The model under review builds one solid part; all positions refer to its coordinate system, in mm. Face numbers are marked on the shaded views. A direction names the side the tool comes from. Give positions to 0.01 mm unless a question says otherwise; leave off trailing zeros. Order: outer loops, then holes, each group sorted by start corner. A loop starts at its lowest first (then second) coordinate and runs counter-clockwise, first axis right, second up.
```python
from build123d import *

# Parameters (mm, degrees)
EXTRUDE_1_DEPTH             = 25
CHAMFER_5_SIZE              = 2.5
SKETCH_6_W                  = 20.2
SKETCH_6_H                  = 41.891303575
CUT_EXTRUDE_2_DEPTH         = 7.6
SKETCH_7_R                  = 5.25
SKETCH_7_R_2                = 4.1
CUT_EXTRUDE_3_DEPTH         = 76.352903063
SKETCH_8_W                  = 20.2
SKETCH_8_H                  = 8.585894888
CUT_EXTRUDE_4_DEPTH         = 5.1
FILLET_2_R                  = 2
CUT_EXTRUDE_5_REACH         = 77.353
SKETCH_10_R                 = 1.5
M3X0_51_D                   = 2.5
M3X0_51_DEPTH               = 3
M3X0_51_TIP                 = 0.751075774
EXTRUDE_3_DEPTH             = 5
FILLET_3_R                  = 2
HOLE_WIZARD_M32_D           = 3.4
HOLE_WIZARD_M32_CBORE_D     = 6.5
HOLE_WIZARD_M32_CBORE_DEPTH = 2.5


with BuildPart() as part:
    # Эскиз1 → Бобышка-Вытянуть1 (new body)
    with BuildSketch(Plane.XY):
        with BuildLine():
            Line((0, 0), (0, 70.5))
            Line((0, 70.5), (-3.6, 70.5))
            ThreePointArc((-3.6, 70.5), (-7.489087297, 68.889087297), (-9.1, 65))
            Line((-9.1, 65), (-9.1, 32))
            ThreePointArc((-9.1, 32), (-8.15059166, 22.302605618), (-5.338421688, 12.97348272))
            Line((-5.338421688, 12.97348272), (0, 0))
        make_face()
    extrude(amount=EXTRUDE_1_DEPTH)

    # Фаска5
    chamfer_5_edges = [part.edges().sort_by_distance(p)[0] for p in [
        (-8.15059166, 22.302605618, 25),
        (-2.669210844, 6.48674136, 25),
        (-1.8, 70.5, 25),
        (-7.489087297, 68.889087297, 25),
        (-1.8, 70.5, 0),
        (-2.669210844, 6.48674136, 0),
        (-9.1, 48.5, 25),
        (-8.15059166, 22.302605618, 0),
        (-9.1, 48.5, 0),
        (-7.489087297, 68.889087297, 0),
    ]]
    chamfer(chamfer_5_edges, length=CHAMFER_5_SIZE)

    # Эскиз6 → Вырез-Вытянуть2 (cut)
    with BuildSketch(Plane(origin=(0, 0, 0), x_dir=(0, 0, -1), z_dir=(1, 0, 0))):
        with Locations((-12.5, 46.054348213)):
            Rectangle(SKETCH_6_W, SKETCH_6_H)
    extrude(amount=-CUT_EXTRUDE_2_DEPTH, mode=Mode.SUBTRACT)

    # Эскиз7 → Вырез-Вытянуть3 (cut, through all)
    with BuildSketch(Plane.ZY.offset(9.1)):
        with Locations(Location((12.5, 35.5, 0), (0, 0, 318.189685104))):
            Circle(SKETCH_7_R)
        with Locations((12.5, 51.5)):
            Circle(SKETCH_7_R_2)
    extrude(amount=-CUT_EXTRUDE_3_DEPTH, mode=Mode.SUBTRACT)

    # Эскиз8 → Вырез-Вытянуть4 (cut)
    with BuildSketch(Plane(origin=(0, 0, 0), x_dir=(0, 0, -1), z_dir=(1, 0, 0))):
        with Locations((-12.5, 20.815748981)):
            Rectangle(SKETCH_8_W, SKETCH_8_H)
    extrude(amount=-CUT_EXTRUDE_4_DEPTH, mode=Mode.SUBTRACT)

    # Скругление2
    fillet_2_edges = [part.edges().sort_by_distance(p)[0] for p in [
        (-3.8, 67, 2.4),
        (-6.35, 25.108696425, 2.4),
        (-6.35, 25.108696425, 22.6),
        (-3.8, 67, 22.6),
        (-2.55, 16.522801537, 22.6),
        (-2.55, 16.522801537, 2.4),
    ]]
    fillet(fillet_2_edges, radius=FILLET_2_R)

    # Эскиз10 → Вырез-Вытянуть5 (cut, up to next)
    with BuildSketch(Plane.ZY.offset(9.1), mode=Mode.PRIVATE) as cut_extrude_5_sk1:
        with Locations((12.5, 22)):
            Circle(SKETCH_10_R)
    cut_extrude_5_tool1 = extrude(cut_extrude_5_sk1.sketch, amount=-CUT_EXTRUDE_5_REACH, mode=Mode.PRIVATE) & part.part
    add(cut_extrude_5_tool1.solids().sort_by_distance((-9.1, 22, 12.5))[0], mode=Mode.SUBTRACT)

    # Отверстие обработанное метчиком M3x0.51
    with Locations(Plane(origin=(0, 0, 0), x_dir=(0, 0, -1), z_dir=(1, 0, 0))):
        with Locations((-12.5, 12)):
            Hole(M3X0_51_D / 2, depth=M3X0_51_DEPTH)
            with Locations((0, 0, -(M3X0_51_DEPTH + M3X0_51_TIP / 2))):  # 118° drill point
                Cone(0, M3X0_51_D / 2, M3X0_51_TIP, mode=Mode.SUBTRACT)

    # Эскиз22 → Бобышка-Вытянуть3 (add)
    with BuildSketch(Plane(origin=(-7.6, 0, 0), x_dir=(0, 0, -1), z_dir=(1, 0, 0))):
        with BuildLine():
            Line((-17.5, 63), (-17.5, 67))
            Line((-17.5, 67), (-7.5, 67))
            Line((-7.5, 67), (-7.5, 63))
            ThreePointArc((-7.5, 63), (-12.5, 58), (-17.5, 63))
        make_face()
    extrude(amount=EXTRUDE_3_DEPTH)

    # Скругление3
    fillet_3_edges = [part.edges().sort_by_distance(p)[0] for p in [
        (-5.1, 67, 7.5),
        (-5.1, 67, 17.5),
    ]]
    fillet(fillet_3_edges, radius=FILLET_3_R)

    # Цековка для винта с внутренним шестигранником M32 (through all)
    with Locations(Plane.ZY.offset(9.1)):
        with Locations((12.5, 63)):
            CounterBoreHole(HOLE_WIZARD_M32_D / 2, HOLE_WIZARD_M32_CBORE_D / 2, HOLE_WIZARD_M32_CBORE_DEPTH)


solid = part.part
```
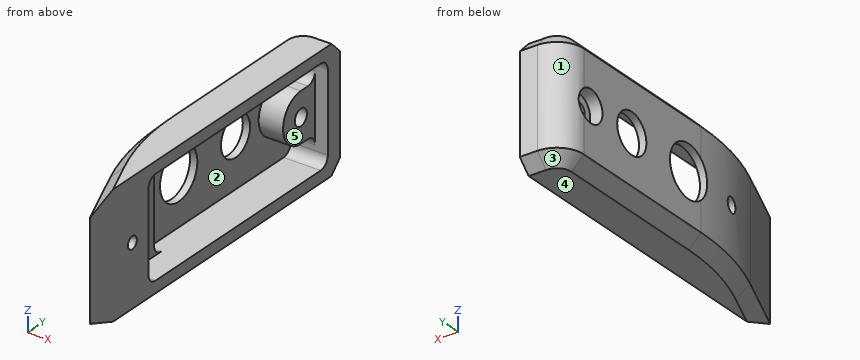
Item 1: For line 1 (Z direction, x = -1.25, y = 34); line 2 (X direction, y = 64.5, z = 4.25); line 3 (Y direction, x = -4.75, z = 4.25), list the stretches that pass through material, from the lowest coordinate up.
Values found:
line 1: z = 0 to 2.4, 22.6 to 25
line 2: x = -9.1 to -7.6
line 3: y = 11.54 to 16.53, 66.99 to 70.38
Item 2: Take a section at A-A (y = 51.5). Give the boundary of the cut face in (x, z), and give its area (3 significant figures).
Values found:
outline: (-9.1, 2.5) - (-6.6, 0) - (0, 0) - (0, 2.4) - (-7.6, 2.4) - (-7.6, 8.4) - (-9.1, 8.4) - close; (-9.1, 16.6) - (-7.6, 16.6) - (-7.6, 22.6) - (0, 22.6) - (0, 25) - (-6.6, 25) - (-9.1, 22.5) - close
area: 55.4 mm2
Item 3: Draft analysis for pull direction Z (two halves, no side actions). For the marked faces 1, 2 and 3, state which applies: released by +Z, released by -Z, zero draft, split by the parting line, or undercut.
Values found:
face 1: zero draft
face 2: undercut
face 3: released by -Z
Item 4: Take a section at B-B (y = 35.5). Give the boundary of the cut face in (x, z), and give its area (3 significant figures).
Values found:
outline: (-9.1, 2.5) - (-6.6, 0) - (0, 0) - (0, 2.4) - (-7.6, 2.4) - (-7.6, 7.25) - (-9.1, 7.25) - close; (-9.1, 17.75) - (-7.6, 17.75) - (-7.6, 22.6) - (0, 22.6) - (0, 25) - (-6.6, 25) - (-9.1, 22.5) - close
area: 52.0 mm2
Item 5: For the marked faces 4 and 5, list the 3-axis set-ups (+Z, -Z, +X, -X, +Y, -Y) from which the entire face can be reached by the end or side of a thin tool; tool diameter is ignored.
Values found:
face 4: -Z, +X, -X, +Y, -Y
face 5: +X
Item 6: Clearance check with flat-ended pins moving along their axes: pin 1 Ø8 at (y, z) = (21, 14) entering from -X; pin 2 Ø11.5 at (y, z) = (24, 10) entering from +X; pin 3 Ø4 at (y, z) = (63, 12.5) entering from +X. State where each tip first meets the part, or that it passes through.
Values found:
pin 1: stops at x = -8.61
pin 2: stops at x = -5.1
pin 3: stops at x = -2.6
